from build123d import *

# Parameters (mm, degrees)
F2_R     = 41.5
F0_R     = 35
F6_DEPTH = 27.5
F7_R     = 33.5
F8_DEPTH = 53


with BuildPart() as f3:
    # F2 (on offset) → F3 section 0
    with BuildSketch(Plane.XY.offset(75)):
        Circle(F2_R)
    # F0 (on Top) → F3 section 1
    with BuildSketch(Plane.XY):
        Circle(F0_R)
    loft()

    # F5 (on Front) → F6 (cut, symmetric)
    with BuildSketch(Plane.XZ):
        Polygon((32.979961, 75), (37.831545, 51.901187), (40.54823, 51.901187), (42.30484, 75), align=None)
    extrude(amount=F6_DEPTH, both=True, mode=Mode.SUBTRACT)

    # F7 (on Top) → F8 (cut)
    with BuildSketch(Plane.XY):
        Circle(F7_R)
    extrude(amount=F8_DEPTH, mode=Mode.SUBTRACT)


solid = f3.part
Input: part model. Units: mm. Frame: model coordinates. A direction names the side the tool comes from. Coordinates: 2 decimals unless noted, no trailing zeros. Loops run counter-clockwise (first coordinate to the right, second up) from the corner with the lowest first, then second, coordinate; pieces in that order, holes last.
(1) Section B-B on z = 39. Return the cut outline in (x, y).
(2) Material intervals for probe 1 along Z at (x, y) = (17.5, 1); probe 2 along Y at (x, z) = (0, 19.5); probe 3 along Y at (x, z) = (19, 49), sorted ascending.
(3) Pull-direction query (Y, two-part tool) for faces 1 (the face through (34.833, -0.353, 66.179)), 2 (the face through (-37.446, 1.648, 28.642)), 3 (the face through (-7.262, -32.703, 26.129)); classes: released by +Y, released by -Y, zero draft, split by the parting line, or undercut.
(4) Set-up query: faces 4 (the face through (-5, 1, 75)), 5 (the face through (0, 0, 53)). Return all of +Z, -Z, +X, -X, +Y, -Y with unobstructed straight access to the full face (end or side cutting, diameter ignored); none if empty.
(5) Section D-D on z = 58. Return the cut outline in (x, y).
(6) Section A-A on x = 0. Return the cut outline in (y, z), then the cut area to 3 significant figures.
(7) Section C-C on z = 18. Return the cut outline in (x, y).
(8) First-contact query: pin 1 Ø8 at (x, z) = (-10, 52) entering from -Y; pin 2 Ø1.3 at (x, y) = (39, 2) entering from +Z; pin 3 Ø6 at (y, z) = (-10.5, 47) entering from -X. Flat tips, straight axial feed; report the tip coordinate or a pass-through.
Data:
1. outline: circle Ø76.76 at (0, 0); hole circle Ø67 at (0, 0)
2. probe 1: z = 53 to 75
2. probe 2: y = -36.69 to -33.5, 33.5 to 36.69
2. probe 3: y = -34.34 to -27.59, 27.59 to 34.34
3. face 1: zero draft
3. face 2: split by the parting line
3. face 3: undercut
4. face 4: +Z, +X, -X, +Y, -Y
4. face 5: -Z
5. outline: (36.55, -16.32) - (36.55, 16.32) arc R40.03 ccw (long way) to start
6. outline: (-41.5, 75) - (-35, 0) - (-33.5, 0) - (-33.5, 53) - (33.5, 53) - (33.5, 0) - (35, 0) - (41.5, 75) - close
6. area: 2,190 mm2
7. outline: circle Ø73.12 at (0, 0); hole circle Ø67 at (0, 0)
8. pin 1: stops at y = -39.14
8. pin 2: stops at z = 51.9
8. pin 3: stops at x = -38.4
